Here's how the part is built. I have some questions about the finished solid (model axes, mm). A direction names the side the tool comes from. Coordinates: 2 decimals unless noted, no trailing zeros. Write each loop counter-clockwise with the first axis right and the second up, starting at its lowest first coordinate (ties: lowest second). Pieces come first, ordered by that corner, then holes.
Autodesk Inventor part; units mm, degrees
ref_plane "YZ Plane" through (0, 0, 0) normal (1, 0, 0) x (0, 1, 0)
ref_plane "XZ Plane" through (0, 0, 0) normal (0, 1, 0) x (-1, 0, 0)
ref_plane "XY Plane" through (0, 0, 0) normal (0, 0, 1) x (1, 0, 0)
sketch "Sketch1" plane through (0, 0, 0) normal (0, 0, 1) x (1, 0, 0)
  circle A0 centre (0, 0) radius 8
  dimension "d0" = 16
extrude "Extrusion1" add sketch "Sketch1" along normal blind 32
sketch "Sketch2" plane through (0, 0, 0) normal (0, 0, -1) x (-1, 0, 0)
  line L0 (0, 10.9) -> (9.4397, 5.45)
  line L1 (9.4397, 5.45) -> (9.4397, -5.45)
  line L2 (9.4397, -5.45) -> (0, -10.9)
  line L3 (0, -10.9) -> (-9.4397, -5.45)
  line L4 (-9.4397, -5.45) -> (-9.4397, 5.45)
  line L5 (-9.4397, 5.45) -> (0, 10.9)
  point P0 (0, 0)
  point P1 (0, 0)
  dimension "d3" = 21.8
extrude "Extrusion2" add sketch "Sketch2" against normal blind 1.5
sketch "Sketch3" plane through (0, 0, 0) normal (0, 0, -1) x (-1, 0, 0)
  circle A0 centre (0, 0) radius 9
  dimension "d6" = 18
extrude "Extrusion3" add sketch "Sketch3" along normal blind 1
sketch "Sketch4" plane through (0, 0, -1) normal (0, 0, -1) x (-1, 0, 0)
  circle A0 centre (0, 0) radius 6.3
  dimension "d9" = 12.6
extrude "Extrusion4" cut sketch "Sketch4" against normal blind 1
sketch "Sketch5" plane through (0, 0, 0) normal (0, 0, -1) x (-1, 0, 0)
  circle A0 centre (0, 0) radius 5.6
  dimension "d12" = 11.2
extrude "Extrusion5" cut sketch "Sketch5" against normal blind 0.5
sketch "Sketch6" plane through (0, 0, -1) normal (0, 0, -1) x (-1, 0, 0)
  circle A0 centre (0, 0) radius 7
  dimension "d15" = 14
extrude "Extrusion6" cut sketch "Sketch6" against normal blind 0.5
properties part number "16mmToggleButton"
1. If I drill on line 1 (Y direction, x = 0, z = -0.65); line 2 (Y direction, x = 0, z = 0.2); line 3 (Z direction, x = 5, y = -4.5), over which ranges is the centre line in solid material (lowest first)?
2. I want a section at B-B (x = 4.25). List the corners of the cut face in (y, z) for me.
3. For pin 1 Ø1.5 at (y, z) = (6.5, 26) entering from -X; pin 2 Ø4 at (x, y) = (-2.5, -1) entering from -Z; pin 3 Ø3 at (x, z) = (3, 22) entering from -Y, each with a flat end and sliding along its axis, tell me the tip position at first contact or that it passes through.
4. On a 3-axis mill with a long thin cutter (end or side, diameter ignored), from which of +Z, -Z, +X, -X, +Y, -Y can I reach the whole of each face in a straight line? I mean faces 4 (the face through (-1.73, 7.81, 16.54)), 5 (the face through (0, 0, 32)), 6 (the face through (5, -3.83, -0.25)). Say none if no direction works.
5. I want a section at C-C (z = 11.5). List the corners of the cut face in (x, y) for me.
6. I want a section at D-D (y = -8.5). List the corners of the cut face in (x, z) for me.
7. I want a section at A-A (y = 0). List the corners of the cut face in (x, z) for me.
8. Thinking about a two-plate mould opening in X: for faces 1 (the face through (9.44, 0, 1)), 2 (the face through (-9.44, 0, 1)), 3 (the face through (5.595, 0.246, 0.246)), which applies, pulls with the +X half, pulls with the -X half, needs draft (parallel to the pull), parting line crosses it, or undercut?
Response values:
1. line 1: y = -9 to -7, 7 to 9
1. line 2: y = -10.9 to -5.6, 5.6 to 10.9
1. line 3: z = -0.5 to 32
2. outline: (-8.45, 0) - (-7.93, 0) - (-7.93, -1) - (-5.56, -1) - (-5.56, -0.5) - (-4.65, -0.5) - (-4.65, 0) - (-3.65, 0) - (-3.65, 0.5) - (3.65, 0.5) - (3.65, 0) - (4.65, 0) - (4.65, -0.5) - (5.56, -0.5) - (5.56, -1) - (7.93, -1) - (7.93, 0) - (8.45, 0) - (8.45, 1.5) - (6.78, 1.5) - (6.78, 32) - (-6.78, 32) - (-6.78, 1.5) - (-8.45, 1.5) - close
3. pin 1: stops at x = -5.56
3. pin 2: stops at z = 0.5
3. pin 3: stops at y = -7.86
4. face 4: +Z
4. face 5: +Z, +X, -X, +Y, -Y
4. face 6: -Z
5. outline: circle Ø16 at (0, 0)
6. outline: (-4.16, 0) - (-2.96, 0) - (-2.96, -1) - (2.96, -1) - (2.96, 0) - (4.16, 0) - (4.16, 1.5) - (-4.16, 1.5) - close
7. outline: (-9.44, 0) - (-9, 0) - (-9, -1) - (-7, -1) - (-7, -0.5) - (-6.3, -0.5) - (-6.3, 0) - (-5.6, 0) - (-5.6, 0.5) - (5.6, 0.5) - (5.6, 0) - (6.3, 0) - (6.3, -0.5) - (7, -0.5) - (7, -1) - (9, -1) - (9, 0) - (9.44, 0) - (9.44, 1.5) - (8, 1.5) - (8, 32) - (-8, 32) - (-8, 1.5) - (-9.44, 1.5) - close
8. face 1: pulls with the +X half
8. face 2: pulls with the -X half
8. face 3: undercut
